Input: dimensioned drawing with shaded views. Units: mm. Origin: part minimum x, y, z. A direction names the side the tool comes from. Round coordinates to 2 decimals unless told otherwise and drop trailing zeros. Loops run counter-clockwise (first coordinate to the right, second up) from the corner with the lowest first, then second, coordinate; pieces in that order, holes last. Notation, with made-up numbers: M 13,41.25 L 63,41.25 A20 ccw 63,54.25 Z; hole C -18,49 d8. An arc over 180 degrees is marked long. Use one line per item in the form item = value. Start each with the question number.
Q1. Section query B-B, the plane x = 4.25. Output: boundary loops of the cut face in (y, z), and give its area (3 significant figures).
Q2. Section query A-A, the plane y = 1.5. Output: boundary loops of the cut face in (x, z).
Q3. Access query for the marked faces 1 and 2. Directions: +Z, -Z, +X, -X, +Y, -Y. A direction counts if a zero-diameter tool reaches every point of the face in a straight line with its end or side. Return the directions, or none.
Q4. Ray query, line 1 along Y through (x, z) = (5.25, 2.4); line 2 along Y through (x, z) = (7, 2.1); line 3 along X through (y, z) = (2.15, 0.4). Return the intervals inside material, ascending.
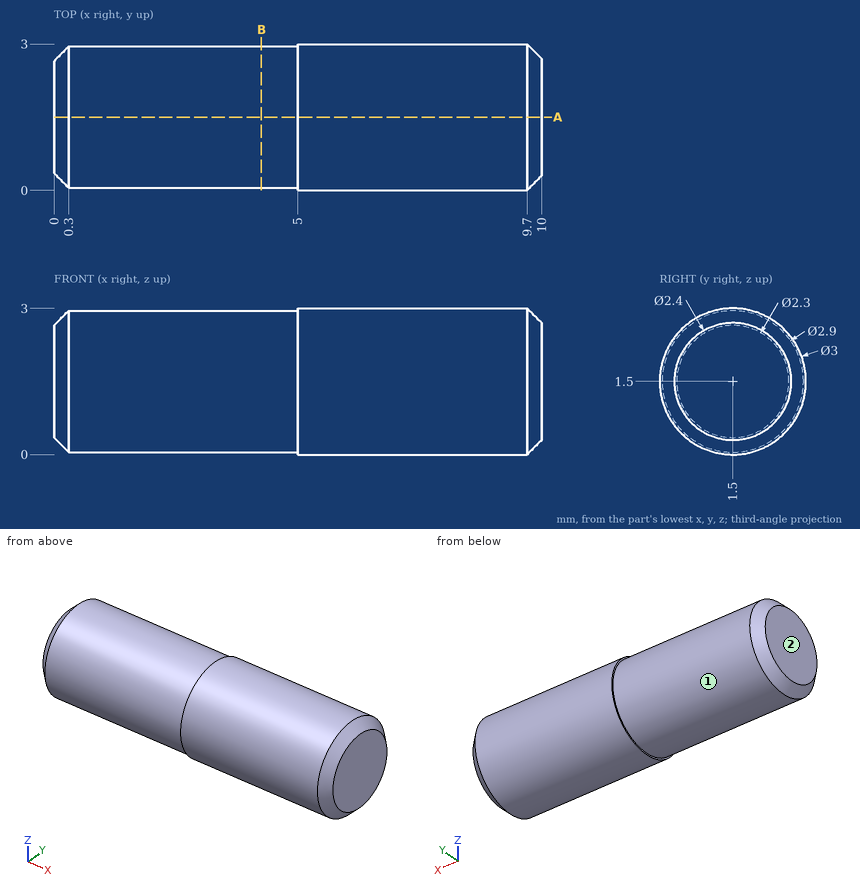
Results found:
q1.outline = C 1.5,1.5 d2.9
q1.area = 6.61 mm²
q2.outline = M 0,0.35 L 0.3,0.05 L 5,0.05 L 5,0 L 9.7,0 L 10,0.3 L 10,2.7 L 9.7,3 L 5,3 L 5,2.95 L 0.3,2.95 L 0,2.65 Z
q3.face_1 = -X
q3.face_2 = +Z, -Z, -X, +Y, -Y
q4.line_1 = 0.3 to 2.7
q4.line_2 = 0.13 to 2.87
q4.line_3 = 0.13 to 9.92
